from build123d import *

# Parameters (mm, degrees)
SKETCH1_R           = 6.5
BOSS_EXTRUDE1_DEPTH = 18
SKETCH2_R           = 5
CUT_EXTRUDE1_DEPTH  = 4
CUT_EXTRUDE2_DEPTH  = 12
CHAMFER1_SIZE       = 1
CHAMFER1_SIZE2      = 0.577350269


with BuildPart() as part:
    # Sketch1 → Boss-Extrude1 (new body)
    with BuildSketch(Plane(origin=(0, 0, 0), x_dir=(1, 0, 0), z_dir=(0, 1, 0))):
        with Locations(Location((0, 0, 0), (0, 0, 270))):
            Circle(SKETCH1_R)
    extrude(amount=BOSS_EXTRUDE1_DEPTH)

    # Sketch2 → Cut-Extrude1 (cut)
    with BuildSketch(Plane.XZ):
        with Locations(Location((0, 0, 0), (0, 0, 270))):
            Circle(SKETCH2_R)
    extrude(amount=-CUT_EXTRUDE1_DEPTH, mode=Mode.SUBTRACT)

    # Sketch3 → Cut-Extrude2 (cut)
    with BuildSketch(Plane.XZ.offset(-4)):
        with BuildLine():
            Line((-1.732055507, -2.57098886), (3.04828024, -0.563903873))
            ThreePointArc((3.04828024, -0.563903873), (-1.200087257, 2.858284551), (-1.732055507, -2.57098886))
        make_face()
    extrude(amount=-CUT_EXTRUDE2_DEPTH, mode=Mode.SUBTRACT)

    # Chamfer1
    chamfer1_edges = [part.edges().sort_by_distance(p)[0] for p in [
        (0, 0, 5),
    ]]
    chamfer1_side = [part.faces().sort_by_distance(p)[0] for p in [
        (0, 2, 5),
    ]]
    chamfer(chamfer1_edges, length=CHAMFER1_SIZE, length2=CHAMFER1_SIZE2, reference=chamfer1_side[0])


solid = part.part
For this review, take the finished solid that the model builds, in its own axes (mm). A direction names the side the tool comes from. Round coordinates to 2 decimals unless told otherwise and drop trailing zeros. Write each loop counter-clockwise with the first axis right and the second up, starting at its lowest first coordinate (ties: lowest second). Pieces come first, ordered by that corner, then holes. Notation, with made-up numbers: (2.5, -10) - (28.5, -10) arc R8 ccw to (28.5, -1) - close; hole circle Ø5 at (51, 59.25). An arc over 180 degrees is marked (long way). Write item = value, one per line. Start each with the question number.
1. Consider section B-B on x = 0. State the section outline as (y, z) points, plus the area to 3 significant figures.
2. Wall thickness on L1, parallel to X at y = 12, z = 0; L2, parallel to X at y = 1.6, z = 0; L3, parallel to Y at x = -2.25, z = 1.5: over which ranges is each line inside the solid? List them lowest first.
3. Consider section A-A on z = 0. State the section outline as (x, y) points, plus the area to 3 significant figures.
4. Draft analysis for pull direction Z (two halves, no side actions). For faces 3 (the face through (0, 18, 0)), 4 (the face through (0, 16, 0)), 5 (the face through (-3.955, 8.874, -5.158)), state which applies: released by +Z, released by -Z, zero draft, split by the parting line, or undercut.
5. Consider section C-C on y = 13. State the section outline as (x, z) points, plus the area to 3 significant figures.
6. For faces 1 (the face through (0.625, 9.916, -1.581)), 2 (the face through (5, 0, 3)), list the 3-axis set-ups (+Z, -Z, +X, -X, +Y, -Y) from which the entire face can be reached by the end or side of a thin tool; tool diameter is ignored.
7. For pin 1 Ø1.5 at (y, z) = (14, 4.5) entering from +X; pin 2 Ø1.5 at (x, z) = (1, 4) entering from -Y; pin 3 Ø1.5 at (x, y) = (-4, 7.5) entering from +Z, all flat-tipped, find the tip position at first contact; note any pin that passes through.
Evaluation:
q1.outline = (0, -6.5) - (18, -6.5) - (18, 6.5) - (0, 6.5) - (0, 5.58) - (1, 5) - (4, 5) - (4, 3.1) - (16, 3.1) - (16, -1.84) - (4, -1.84) - (4, -5) - (1, -5) - (0, -5.58) - close
q1.area = 134 mm2
q2.L1 = -6.5 to -3.1, 3.1 to 6.5
q2.L2 = -6.5 to -5, 5 to 6.5
q2.L3 = 16 to 18
q3.outline = (-6.5, 0) - (-5.58, 0) - (-5, 1) - (-5, 4) - (-3.1, 4) - (-3.1, 16) - (3.1, 16) - (3.1, 4) - (5, 4) - (5, 1) - (5.58, 0) - (6.5, 0) - (6.5, 18) - (-6.5, 18) - close
q3.area = 119 mm2
q4.face_3 = zero draft
q4.face_4 = undercut
q4.face_5 = split by the parting line
q5.outline = circle Ø13 at (0, 0); hole (-1.73, -2.57) - (3.05, -0.56) arc R3.1 ccw (long way) to start
q5.area = 108 mm2
q6.face_1 = -Y
q6.face_2 = +Z, -Z, +X, -X, -Y
q7.pin_1 = 5.31
q7.pin_2 = 4
q7.pin_3 = 5.63
